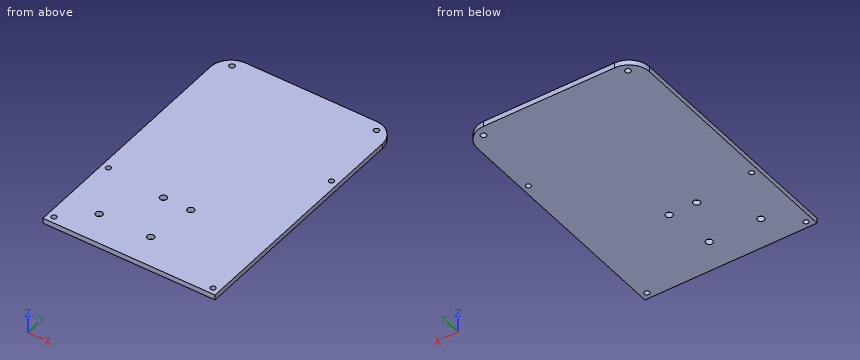
from build123d import *

# Parameters (mm, degrees)
SKETCH1_W           = 100
SKETCH1_H           = 150.5
BOSS_EXTRUDE1_DEPTH = 3
SKETCH2_R           = 1.5
CUT_EXTRUDE1_DEPTH  = 3
SKETCH3_R           = 2
CUT_EXTRUDE2_DEPTH  = 3
FILLET1_R           = 12
SKETCH4_R           = 1.6
CUT_EXTRUDE3_DEPTH  = 10


with BuildPart() as part:
    # Sketch1 → Boss-Extrude1 (new body)
    with BuildSketch(Plane.XY):
        with Locations((-110.534791728, -38.017977095)):
            Rectangle(SKETCH1_W, SKETCH1_H)
    extrude(amount=BOSS_EXTRUDE1_DEPTH)

    # Sketch2 → Cut-Extrude1 (cut)
    with BuildSketch(Plane.XY.offset(3)):
        with Locations((-156.784791728, -109.517977095)):
            Circle(SKETCH2_R)
        with Locations((-64.284791728, -109.517977095)):
            Circle(SKETCH2_R)
        with Locations((-64.284791728, -11.517977095)):
            Circle(SKETCH2_R)
        with Locations((-156.784791728, -64.517977095)):
            Circle(SKETCH2_R)
    extrude(amount=-CUT_EXTRUDE1_DEPTH, mode=Mode.SUBTRACT)

    # Sketch3 → Cut-Extrude2 (cut)
    with BuildSketch(Plane.XY.offset(3)):
        with Locations((-140.534791728, -95.267977095)):
            Circle(SKETCH3_R)
        with Locations((-110.534791728, -95.267977095)):
            Circle(SKETCH3_R)
        with Locations((-106.534791728, -67.767977095)):
            Circle(SKETCH3_R)
        with Locations((-122.534791728, -67.767977095)):
            Circle(SKETCH3_R)
    extrude(amount=-CUT_EXTRUDE2_DEPTH, mode=Mode.SUBTRACT)

    # Fillet1
    fillet1_edges = [part.edges().sort_by_distance(p)[0] for p in [
        (-160.534791728, 37.232022905, 1.5),
        (-60.534791728, 37.232022905, 1.5),
    ]]
    fillet(fillet1_edges, radius=FILLET1_R)

    # Sketch4 → Cut-Extrude3 (cut)
    with BuildSketch(Plane.XY.offset(3)):
        with Locations((-152.534791728, 31.732022905)):
            Circle(SKETCH4_R)
        with Locations((-68.534791728, 31.732022905)):
            Circle(SKETCH4_R)
    extrude(amount=-CUT_EXTRUDE3_DEPTH, mode=Mode.SUBTRACT)


solid = part.part
Geometry: final body of the model. Coordinates: model frame, mm. Coordinates: 2 decimals unless noted, no trailing zeros. Loops run counter-clockwise (first coordinate to the right, second up) from the corner with the lowest first, then second, coordinate; pieces in that order, holes last. Notation, with made-up numbers: (-10.5, -37.5) - (26.5, -37.5) arc R23 cw to (26.5, 1.5) - close; hole circle Ø7 at (69, 73). An arc over 180 degrees is marked (long way). Put each result on its own line as item: value. Start each with the question number.
Q1. Cut plane A-A, the plane x = -140. Return loops of the section in (y, z), and give its area (3 significant figures).
Q2. Line query: line 1 (Y direction, x = -110.5, z = 2.1); line 2 (X direction, y = -65, z = 0.95); line 3 (Y direction, x = -142, z = 2.9). Output: solid intervals per line, ascending.
Q3. Pin query (flat end, axial travel): pin 1 Ø1.8 at (x, y) = (-156.78, -64.52) entering from -Z. Return the tip coordinate at first contact, or that it passes through.
Filled sheet:
1. outline: (-113.27, 0) - (-97.2, 0) - (-97.2, 3) - (-113.27, 3) - close; (-93.34, 0) - (37.23, 0) - (37.23, 3) - (-93.34, 3) - close
1. area: 440 mm²
2. line 1: -113.27 to -97.27, -93.27 to 37.23
2. line 2: -160.53 to -158.21, -155.36 to -60.53
2. line 3: -113.27 to -96.63, -93.91 to 37.23
3. pin 1: through
